Could you check a few things on this drawing? It's one solid part, dimensions in mm from its lowest x, y, z. A direction names the side the tool comes from. Round coordinates to 2 decimals unless told otherwise and drop trailing zeros. Loops run counter-clockwise (first coordinate to the right, second up) from the corner with the lowest first, then second, coordinate; pieces in that order, holes last. Notation, with made-up numbers: (53, -30) -> (66, -30) arc R21 cw to (66, -11) -> close; hole circle Ø10 at (-25, 4.5). An arc over 180 degrees is marked (long way). Put each result on its own line as item: value. Start each with the question number.
1. Which directions (+Z, -Z, +X, -X, +Y, -Y) give clear straight access to the entire face, cutting with the end or side of a thin tool? Please do the marked faces 4 and 5.
2. If we mould it in two halves opening along Y, with no side actions, what happens to the marked faces 1, 2 and 3? For each: pulls with the +Y half, pulls with the -Y half, needs draft (parallel to the pull), parting line crosses it, or undercut.
3. Imagine slicing it at D-D, the plane z = 4.4. Please give me the cut outline in (x, y).
4. I'm going to push flat-ended pins straight in: P1, Ø5, axis at x = 14, y = 28, coming from the -Z side; P2, Ø1, axis at y = 7, z = 1, coming from the -X side; P3, Ø1, axis at y = 29, z = 3, coming from the -X side; P4, Ø3, axis at x = 20, y = 13.5, coming from the -Z side. Where does each tip first touch, or does it pass through?
5. I need wall thicknesses on line 1 (Y direction, x = 16, z = 1.35); line 2 (Y direction, x = 7.5, z = 4.75); line 3 (X direction, y = 21, z = 1.4). Which ranges of each line are inside material? Lowest first, please. Write a range as [from, to].
6. Imagine slicing it at A-A, the plane y = 16. Please give me the cut outline in (x, z), and give its area (4 significant figures).
7. Imagine slicing it at C-C, the plane z = 1.1. Please give me the cut outline in (x, y).
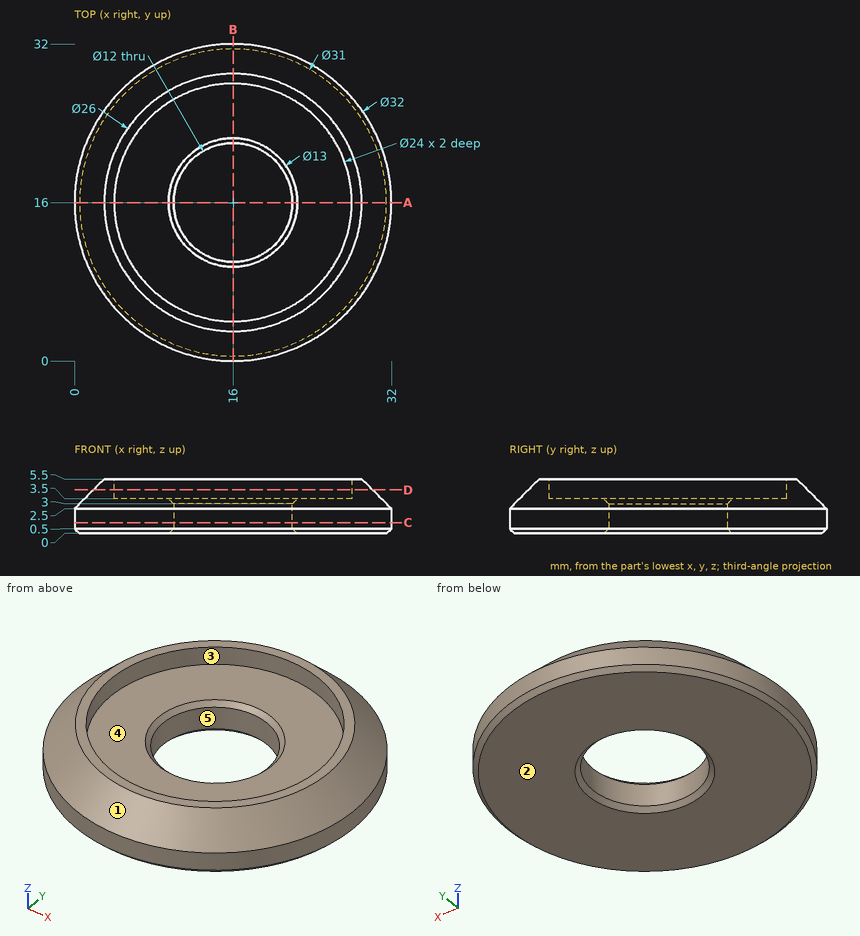
Entries:
1. face 4: +Z
1. face 5: +Z, -Z
2. face 1: parting line crosses it
2. face 2: needs draft
2. face 3: undercut
3. outline: circle Ø28.2 at (16, 16); hole circle Ø24 at (16, 16)
4. P1: z = 0
4. P2: x = 2.44
4. P3: x = 6.43
4. P4: z = 0.28
5. line 1: [0, 10], [22, 32]
5. line 2: [5.19, 7.53], [24.47, 26.81]
5. line 3: [0.8, 12.68], [19.32, 31.2]
6. outline: (0, 0.5) -> (0.5, 0) -> (9.5, 0) -> (10, 0.5) -> (10, 3) -> (9.5, 3.5) -> (4, 3.5) -> (4, 5.5) -> (3, 5.5) -> (0, 2.5) -> close; (22, 0.5) -> (22.5, 0) -> (31.5, 0) -> (32, 0.5) -> (32, 2.5) -> (29, 5.5) -> (28, 5.5) -> (28, 3.5) -> (22.5, 3.5) -> (22, 3) -> close
6. area: 76.25 mm^2
7. outline: circle Ø32 at (16, 16); hole circle Ø12 at (16, 16)
